from build123d import *

# Parameters (mm, degrees)
SKETCH_1_W          = 30
SKETCH_1_H          = 16
EXTRUDE_1_DEPTH     = 2.5
SKETCH_3_R          = 1.65
CUT_EXTRUDE_1_DEPTH = 2.5
SKETCH_4_W          = 5.8
SKETCH_4_H          = 11
CUT_EXTRUDE_2_DEPTH = 2.5
SKETCH_5_W          = 3
SKETCH_5_H          = 11
EXTRUDE_2_DEPTH     = 11
SKETCH_6_R          = 1.65
CUT_EXTRUDE_3_DEPTH = 27.135416584
CUT_EXTRUDE_4_DEPTH = 21.248456731
CHAMFER_1_SIZE      = 2
FILLET_1_R          = 1
FILLET_2_R          = 0.5
CUT_EXTRUDE_6_DEPTH = 21.248456731


with BuildPart() as part:
    # 草图1 → 凸台-拉伸1 (new body)
    with BuildSketch(Plane(origin=(0, 0, 0), x_dir=(1, 0, 0), z_dir=(0, 1, 0))):
        Rectangle(SKETCH_1_W, SKETCH_1_H)
    extrude(amount=EXTRUDE_1_DEPTH)

    # 草图3 → 切除-拉伸1 (cut)
    with BuildSketch(Plane(origin=(0, 2.5, 0), x_dir=(1, 0, 0), z_dir=(0, 1, 0))):
        with Locations(Location((-12, 5, 0), (0, 0, 270))):
            Circle(SKETCH_3_R)
        with Locations(Location((12, 5, 0), (0, 0, 90))):
            Circle(SKETCH_3_R)
        with Locations(Location((12, -5, 0), (0, 0, 270))):
            Circle(SKETCH_3_R)
        with Locations(Location((-12, -5, 0), (0, 0, 90))):
            Circle(SKETCH_3_R)
        with Locations(Location((0, 5, 0), (0, 0, 270))):
            Circle(SKETCH_3_R)
    extrude(amount=-CUT_EXTRUDE_1_DEPTH, mode=Mode.SUBTRACT)

    # 草图4 → 切除-拉伸2 (cut)
    with BuildSketch(Plane(origin=(0, 2.5, 0), x_dir=(1, 0, 0), z_dir=(0, 1, 0))):
        with Locations((0, 2.5)):
            Rectangle(SKETCH_4_W, SKETCH_4_H)
    extrude(amount=-CUT_EXTRUDE_2_DEPTH, mode=Mode.SUBTRACT)

    # 草图5 → 凸台-拉伸2 (add)
    with BuildSketch(Plane(origin=(0, 2.5, 0), x_dir=(1, 0, 0), z_dir=(0, 1, 0))):
        with Locations((-4.4, 2.5)):
            Rectangle(SKETCH_5_W, SKETCH_5_H)
        with Locations((4.4, 2.5)):
            Rectangle(SKETCH_5_W, SKETCH_5_H)
    extrude(amount=EXTRUDE_2_DEPTH)

    # 草图6 → 切除-拉伸3 (cut, through all)
    with BuildSketch(Plane.ZY.offset(5.9)):
        with Locations((-2.5, 8)):
            Circle(SKETCH_6_R)
    extrude(amount=-CUT_EXTRUDE_3_DEPTH, mode=Mode.SUBTRACT)

    # 草图7 → 切除-拉伸4 (cut, through all)
    with BuildSketch(Plane(origin=(0, 2.5, 0), x_dir=(1, 0, 0), z_dir=(0, 1, 0))):
        Polygon((-15, 2), (-3, -8), (-15, -8), align=None)
        Polygon((3, -8), (15, -8), (15, 2), align=None)
    extrude(amount=-CUT_EXTRUDE_4_DEPTH, mode=Mode.SUBTRACT)

    # 倒角1
    chamfer_1_edges = [part.edges().sort_by_distance(p)[0] for p in [
        (-4.4, 13.5, -8),
        (-4.4, 13.5, 3),
        (4.4, 13.5, 3),
        (4.4, 13.5, -8),
        (-15, 1.25, -8),
        (15, 1.25, -8),
    ]]
    chamfer(chamfer_1_edges, length=CHAMFER_1_SIZE)

    # 圆角1
    fillet_1_edges = [part.edges().sort_by_distance(p)[0] for p in [
        (-2.9, 1.25, 3),
        (2.9, 1.25, 3),
    ]]
    fillet(fillet_1_edges, radius=FILLET_1_R)

    # 圆角2
    fillet_2_edges = [part.edges().sort_by_distance(p)[0] for p in [
        (-2.9, 2.5, 2.5),
        (2.9, 2.5, 2.5),
        (-5.9, 2.5, -2.5),
        (-4.4, 2.5, 3),
        (4.4, 2.5, 3),
        (5.9, 2.5, -2.5),
    ]]
    fillet(fillet_2_edges, radius=FILLET_2_R)

    # 草图8 → 切除-拉伸6 (cut, through all)
    with BuildSketch(Plane(origin=(0, 2.5, 0), x_dir=(1, 0, 0), z_dir=(0, 1, 0))):
        Polygon((-6, -5.5), (6, -5.5), (3, -8), (-3, -8), align=None)
    extrude(amount=-CUT_EXTRUDE_6_DEPTH, mode=Mode.SUBTRACT)


solid = part.part
Geometry check sheet. Reference: the model listing, model coordinates, mm. A direction names the side the tool comes from. Round coordinates to 2 decimals unless told otherwise and drop trailing zeros. Loops run counter-clockwise (first coordinate to the right, second up) from the corner with the lowest first, then second, coordinate; pieces in that order, holes last. Notation, with made-up numbers: (56.25, 34) -> (77.25, 34) arc R16 ccw to (77.25, 56) -> close; hole circle Ø9 at (82, 80.25). An arc over 180 degrees is marked (long way). Answer as a JSON object with one key per item and string values. Group by question number.
Item 1: Cross-section at A-A, the plane y = 12.75. Record the cut outline in (x, z), plus the area to 3 significant figures.
Item 2: Cross-section at C-C, the plane z = 0.5. Record the cut outline in (x, y).
Item 3: Cross-section at B-B, the plane z = -5. Record the cut outline in (x, y).
Item 4: Release check for a two-part mould opening along X. For faces 1 (the face through (-14, 1, -7)), 2 (the face through (-2.9, 7, -4)), 3 (the face through (0, 1, 5.5)) record: pulls with the +X half, pulls with the -X half, needs draft (parallel to the pull), parting line crosses it, or undercut.
Item 5: Depth check by flat-ended pin: pin 1 Ø1 at (y, z) = (11, -3) entering from -X; pin 2 Ø1 at (y, z) = (5.5, 0) entering from +X; pin 3 Ø3 at (x, y) = (-3.5, 7.5) entering from +Z. Enter the tip coordinate at first touch or a pass-through.
Item 6: Cross-section at D-D, the plane x = -12. Record the cut outline in (y, z), plus the area to 3 significant figures.
Item 7: Set-up check for faces 4 (the face through (0, 1, 3)), 5 (the face through (-4.421, 8.496, -0.926)), 6 (the face through (-4, 7, 3)): record each of +Z, -Z, +X, -X, +Y, -Y from which the full face is reachable in a straight line by a thin tool's end or side.
Item 8: Thickness scan on line 1 along X through (y, z) = (0.7, -5); line 2 along X through (y, z) = (4.25, -0.25); line 3 along Y through (x, z) = (8.25, -1). Record the ranges inside material, lowest first.
Determined:
{
 "1": {"outline": "(-5.9, -6.75) -> (-2.9, -6.75) -> (-2.9, 1.75) -> (-5.9, 1.75) -> close; (2.9, -6.75) -> (5.9, -6.75) -> (5.9, 1.75) -> (2.9, 1.75) -> close", "area": "51.0 mm²"},
 "2": {"outline": "(-12, 0) -> (-2.9, 0) -> (-2.9, 13.5) -> (-5.9, 13.5) -> (-5.9, 3) arc R0.5 cw to (-6.4, 2.5) -> (-12, 2.5) -> close; (2.9, 0) -> (12, 0) -> (12, 2.5) -> (6.4, 2.5) arc R0.5 cw to (5.9, 3) -> (5.9, 13.5) -> (2.9, 13.5) -> close"},
 "3": {"outline": "(-15, 0) -> (-13.65, 0) -> (-13.65, 2.5) -> (-15, 2.5) -> close; (-10.35, 0) -> (-2.9, 0) -> (-2.9, 13.5) -> (-5.9, 13.5) -> (-5.9, 3) arc R0.5 cw to (-6.4, 2.5) -> (-10.35, 2.5) -> close; (2.9, 0) -> (10.35, 0) -> (10.35, 2.5) -> (6.4, 2.5) arc R0.5 cw to (5.9, 3) -> (5.9, 13.5) -> (2.9, 13.5) -> close; (13.65, 0) -> (15, 0) -> (15, 2.5) -> (13.65, 2.5) -> close"},
 "4": {"face 1": "pulls with the -X half", "face 2": "undercut", "face 3": "needs draft"},
 "5": {"pin 1": "stops at x = -5.9", "pin 2": "stops at x = 5.9", "pin 3": "stops at z = 3"},
 "6": {"outline": "(0, -8) -> (2.5, -8) -> (2.5, -6.65) -> (0, -6.65) -> close; (0, -3.35) -> (2.5, -3.35) -> (2.5, 0.5) -> (0, 0.5) -> close", "area": "13.0 mm²"},
 "7": {"face 4": "-Z, +Y, -Y", "face 5": "+X, -X", "face 6": "+Z, +X, -X, +Y"},
 "8": {"line 1": "x = -15 to -13.65, -10.35 to -2.9, 2.9 to 10.35, 13.65 to 15", "line 2": "x = -5.9 to -2.9, 2.9 to 5.9", "line 3": "y = 0 to 2.5"}
}
